Design review of the part built by this model. Coordinates are the model's own, in mm. A direction names the side the tool comes from. Round coordinates to 2 decimals unless told otherwise and drop trailing zeros. Loops run counter-clockwise (first coordinate to the right, second up) from the corner with the lowest first, then second, coordinate; pieces in that order, holes last. Notation, with made-up numbers: (35, 87.25) - (56, 87.25) arc R18 cw to (56, 109.25) - close; hole circle Ø8 at (6, -18.75). An arc over 180 degrees is marked (long way). Return JSON: item names as keys, results as strings. Group by question number.
(1) Clearance check with flat-ended pins moving along their axes: pin 1 (2 mm diameter, centred on x = -12, y = -8.5, fed in from -Z); pin 2 (4.5 mm diameter, centred on x = -5, y = 6, fed in from +Z); pin 3 (3 mm diameter, centred on x = -9.5, z = -1.5, fed in from -Y); pin 4 (1.2 mm diameter, centred on x = 7, z = 1, fed in from +Y). State where each tip first meets the part, or that it passes through.
(2) We need section B-B, the plane z = -3. Write out the cut boundary in (x, y), and give its area (3 significant figures).
(3) For faces 1 (the flat face through (-7, -10, 0)), 2 (the flat face through (-7, -6.519, 0)), 3 (the flat face through (-3, -10, 1.5)), 4 (the flat face through (9.5, 1, 0)), 5 (the flat face through (0, 6, 0)), list the 3-axis set-ups (+Z, -Z, +X, -X, +Y, -Y) from which the entire face can be reached by the end or side of a thin tool; tool diameter is ignored.
(4) We need section A-A, the plane x = -8. Write out the cut boundary in (y, z).
(5) Wall thickness on L1, parallel to Y at x = -13.5, z = -2.5; L2, parallel to Z at x = 5.25, y = -2; L3, parallel to Y at x = 8.25, z = -2.5: over which ranges is each line inside the solid? List them lowest first. Write a range as [from, to].
(6) We need section D-D, the plane x = 3. Write out the cut boundary in (y, z).
(7) We need section C-C, the plane y = 3. Write out the cut boundary in (x, z) (3 decimals), and give its area (3 significant figures).
(8) The part is to be moulded in two halves that separate along Z. For faces 6 (the flat face through (-3, 6, 1.5)), 7 (the flat face through (0, 0, 2)), 8 (the cylindrical face through (-11.623, 3.467, 0.071)), say which applies: pulls with the +Z half, pulls with the -Z half, needs draft (parallel to the pull), parting line crosses it, or undercut.
from build123d import *

# Parameters (mm, degrees)
F1_DEPTH  = 5
F2_R      = 1.625
F3_DEPTH  = 25
F4_DEPTH  = 25
F6_DEPTH  = 4
F7_W      = 7
F7_H      = 3
F8_DEPTH  = 4
F9_DEPTH  = 1.5
F11_DEPTH = 7
F13_DEPTH = 25
F14_D     = 5
F14_DEPTH = 20
F14_TIP   = 1.5021515476


with BuildPart() as f1:
    # F0 (on Top) → F1 (new body, symmetric)
    with BuildSketch(Plane.XY):
        Polygon((0, -6.5188171205), (-15, -6.5188171205), (-15, -8.5188171205), (3, -8.5188171205), (3, 4.4811828795), (-15, 4.4811828795), (-15, 2.4811828795), (0, 2.4811828795), (0, 0), align=None)
    extrude(amount=F1_DEPTH, both=True)

    # F2 (on face) → F3 (cut)
    with BuildSketch(Plane.XZ.offset(8.5188171205)):
        with Locations((-10, 0)):
            Circle(F2_R)
    extrude(amount=-F3_DEPTH, mode=Mode.SUBTRACT)

    # F2 (on face) → F4 (cut)
    with BuildSketch(Plane.XZ.offset(8.5188171205)):
        with BuildLine():
            ThreePointArc((-15, 0), (-13.5355339059, 3.5355339059), (-10, 5))
            Line((-10, 5), (-15, 5))
            Line((-15, 5), (-15, 0))
        make_face()
        with BuildLine():
            Line((-15, -5), (-10, -5))
            ThreePointArc((-10, -5), (-13.5355339059, -3.5355339059), (-15, 0))
            Line((-15, 0), (-15, -5))
        make_face()
    extrude(amount=-F4_DEPTH, mode=Mode.SUBTRACT)

    # F5 (on face) → F6 (join)
    with BuildSketch(Plane.XZ.offset(8.5188171205)):
        Polygon((0, 0), (0, 1.5), (-7, 1.5), (-7, -1.5), (0, -1.5), align=None)
    extrude(amount=F6_DEPTH)

    # F7 (on face) → F8 (join)
    with BuildSketch(Plane(origin=(0, 4.4811828795, 0), x_dir=(-1, 0, 0), z_dir=(0, 1, 0))):
        with Locations((3.5, 0)):
            Rectangle(F7_W, F7_H)
    extrude(amount=F8_DEPTH)

    # F9 (add): a face of the model
    f9_faces = [f1.faces().sort_by_distance(p)[0] for p in [
        (3, -2.0188171205, 0),
    ]]
    extrude(f9_faces, amount=F9_DEPTH)

    # F11 (add): a face of the model
    f11_faces = [f1.faces().sort_by_distance(p)[0] for p in [
        (4.5, -2.0188171205, 0),
    ]]
    extrude(f11_faces, amount=F11_DEPTH)

    # F12 (on face) → F13 (cut)
    with BuildSketch(Plane(origin=(0, 0, -5), x_dir=(1, 0, 0), z_dir=(0, 0, -1))):
        Polygon((9.5, -1.7511828795), (9.5, 2.0188171205), (9.5, 5.7888171205), (5.5, 5.7888171205), (5.5, -1.7511828795), align=None)
    extrude(amount=-F13_DEPTH, mode=Mode.SUBTRACT)

    # F14
    with Locations(Plane(origin=(0, 0, 0), x_dir=(0, -1, 0), z_dir=(-1, 0, 0))):
        with Locations((2.0188171205, 0)):
            Hole(F14_D / 2, depth=F14_DEPTH)
            with Locations((0, 0, -(F14_DEPTH + F14_TIP / 2))):  # 118° drill point
                Cone(0, F14_D / 2, F14_TIP, mode=Mode.SUBTRACT)


solid = f1.part
Solutions:
{
 "1": {"pin 1": "z = -4.9", "pin 2": "z = 5", "pin 3": "y = -8.52", "pin 4": "y = 4.48"},
 "2": {"outline": "(-14, -8.52) - (11.5, -8.52) - (11.5, 4.48) - (-14, 4.48) - (-14, 2.48) - (0, 2.48) - (0, -6.52) - (-14, -6.52) - close; hole (5.5, -5.79) - (9.5, -5.79) - (9.5, 1.75) - (5.5, 1.75) - close", "area": "175 mm^2"},
 "3": {"face 1": "+Z, -Z, -X, -Y", "face 2": "+Z, -Z, -X", "face 3": "+Z, +X, -X, -Y", "face 4": "+Z, -Z", "face 5": "+Z, -Z, +X, +Y"},
 "4": {"outline": "(-8.52, -5) - (-6.52, -5) - (-6.52, 5) - (-8.52, 5) - close; (2.48, -5) - (4.48, -5) - (4.48, 5) - (2.48, 5) - close"},
 "5": {"L1": "[-8.52, -6.52], [2.48, 4.48]", "L2": "[-5, -2.5], [2.5, 5]", "L3": "[-8.52, -5.79], [1.75, 4.48]"},
 "6": {"outline": "(-8.52, -5) - (4.48, -5) - (4.48, 5) - (-8.52, 5) - close; hole circle Ø5 at (-2.02, 0)"},
 "7": {"outline": "(-10, -5) - (11.5, -5) - (11.5, 5) - (-10, 5) arc R5 ccw to start; hole circle Ø3.25 at (-10, 0)", "area": "246 mm^2"},
 "8": {"face 6": "pulls with the +Z half", "face 7": "needs draft", "face 8": "undercut"}
}
